Autodesk Inventor part; units mm, degrees
ref_plane "YZ Plane" through (0, 0, 0) normal (1, 0, 0) x (0, 1, 0)
ref_plane "XZ Plane" through (0, 0, 0) normal (0, 1, 0) x (-1, 0, 0)
ref_plane "XY Plane" through (0, 0, 0) normal (0, 0, 1) x (1, 0, 0)
sketch "Sketch1" plane through (0, 0, 0) normal (0, 1, 0) x (-1, 0, 0)
  circle A0 centre (0, 0) radius 1.7
  arc A1 (-3.175, 0) -> (3.175, 0) centre (0, 0) ccw
  line L0 (-3.175, 0) -> (-3.175, 17.399)
  line L1 (3.175, 17.399) -> (3.175, 0)
  arc A2 (3.175, 17.399) -> (-3.175, 17.399) centre (0, 17.399) ccw
  circle A3 centre (0, 10.9474) radius 1.7
  dimension "d0" = 3.4
  dimension "d1" = 6.35
  dimension "d6" = 6.35
  dimension "d8" = 17.399
  dimension "d9" = 3.4
  dimension "d10" = 10.9474
extrude "Extrusion1" add sketch "Sketch1" along normal blind 9
properties part number "Limit switch trigger spacer extension arm"
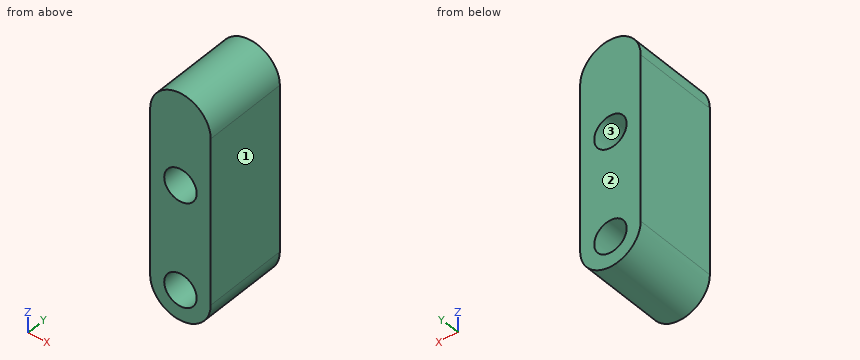
Verification items for the finished model (mm, model axes). Face numbers are marked on the shaded views. Coordinates: 2 decimals unless noted, no trailing zeros. Order: outer loops, then holes, each group sorted by start corner. A loop starts at its lowest first (then second) coordinate and runs counter-clockwise, first axis right, second up. Notation, with made-up numbers: M 55,-36 L 68,-36 A31 cw 68,1 Z; hole C 49,12 d3. An arc over 180 degrees is marked long. One line per item, written item: value. Start each with the question number.
Item 1: Gauge pin test, flat ends, axial feed: pin 1 (3 mm diameter, centred on x = 0, z = 0, fed in from +Y); pin 2 (3 mm diameter, centred on x = -1, y = 3.5, fed in from -Z) (3 decimals). Record the tip position at first contact, or that the pin passes through.
Item 2: Mould release check, pull along X, two halves, no side actions. Record for the marked faces 1, 2 and 3: released by +X, released by -X, zero draft, split by the parting line, or undercut.
Item 3: Sectioned sample at D-D (x = -1). Enter the section's corners in (y, z), then the cut area to 3 significant figures.
Item 4: Scan lines: probe 1 along Z at (x, y) = (0, 5) (3 decimals); probe 2 along Z at (x, y) = (0.25, 8); probe 3 along X at (y, z) = (0.5, -0.75). Record each from-to range of solid material in increasing order.
Item 5: Sectioned sample at C-C (y = 6). Enter the section's corners in (x, z) (3 decimals), then the cut area to 3 significant figures.
Item 6: Sectioned sample at A-A (x = 0). Enter the section's corners in (y, z) (3 decimals), then the cut area to 3 significant figures.
Item 7: Sectioned sample at B-B (z = 0.5). Enter the section's corners in (x, y) (3 decimals), then the cut area to 3 significant figures.
Conclusion:
1. pin 1: passes through
1. pin 2: stops at z = -3.175
2. face 1: released by +X
2. face 2: zero draft
2. face 3: undercut
3. outline: M 0,-3.01 L 9,-3.01 L 9,-1.37 L 0,-1.37 Z; M 0,1.37 L 9,1.37 L 9,9.57 L 0,9.57 Z; M 0,12.32 L 9,12.32 L 9,20.41 L 0,20.41 Z
3. area: 161 mm^2
4. probe 1: z = -3.175 to -1.7, 1.7 to 9.247, 12.647 to 20.574
4. probe 2: z = -3.17 to -1.68, 1.68 to 9.27, 12.63 to 20.56
4. probe 3: x = -3.09 to -1.53, 1.53 to 3.09
5. outline: M -3.175,0 A3.175 ccw 3.175,0 L 3.175,17.399 A3.175 ccw -3.175,17.399 Z; hole C 0,0 d3.4; hole C 0,10.947 d3.4
5. area: 124 mm^2
6. outline: M 0,-3.175 L 9,-3.175 L 9,-1.7 L 0,-1.7 Z; M 0,1.7 L 9,1.7 L 9,9.247 L 0,9.247 Z; M 0,12.647 L 9,12.647 L 9,20.574 L 0,20.574 Z
6. area: 153 mm^2
7. outline: M -3.175,0 L -1.625,0 L -1.625,9 L -3.175,9 Z; M 1.625,0 L 3.175,0 L 3.175,9 L 1.625,9 Z
7. area: 27.9 mm^2
